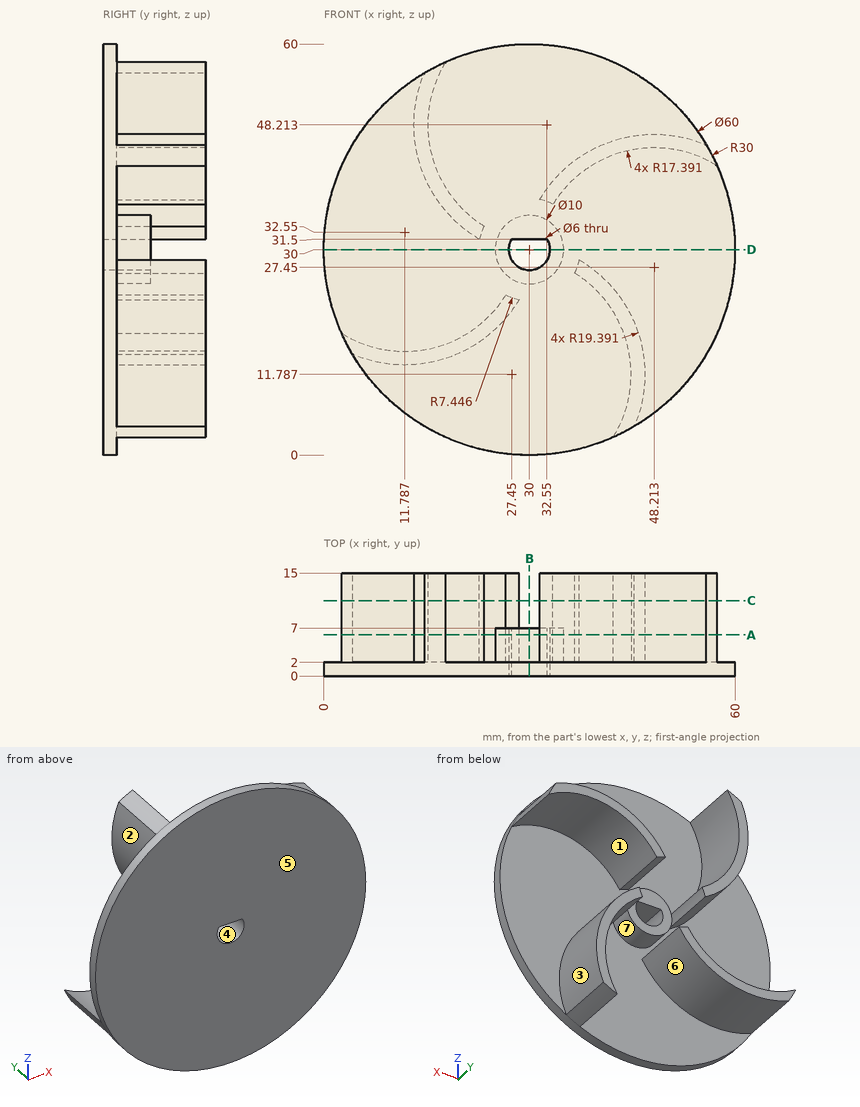
Answer from the drawing. Dimensions are ordinates in mm from the lowest x, y and z of the part. A direction names the side the tool comes from. Coordinates: 2 decimals unless noted, no trailing zeros. Write each loop counter-clockwise with the first axis right and the second up, starting at its lowest first coordinate (ties: lowest second). Pieces come first, ordered by that corner, then holes. Notation, with made-up numbers: (49, -24.75) - (94, -24.75) arc R18 ccw to (94, 1.25) - close; hole circle Ø7 at (-15, 36). An arc over 180 degrees is marked (long way). Return JSON: item names as keys, results as strings.
1. Consider line 1 along Z through (x, y) = (30, 4.75); line 2 along X through (y, z) = (4.75, 30); line 3 along X through (y, z) = (5.5, 28) (1 decimal). Determine where each line is inside the solid, lowest interval first.
Final values:
{"line 1": "25 to 27, 31.5 to 35", "line 2": "25 to 27, 33 to 35", "line 3": "25.4 to 27.8, 32.2 to 34.6, 37.2 to 38.1"}
2. Each of these flat-tipped pins is pushed along its axis until it touches: pin 1 Ø8 at (x, y) = (49.5, 7.5) entering from +Z; pin 2 Ø6 at (x, y) = (23, 12) entering from +Z (1 decimal); pin 3 Ø3 at (y, z) = (13, 16.5) entering from +X. Where does it stop, or does it pass through?
Final values:
{"pin 1": "z = 46.84", "pin 2": "z = 36.2", "pin 3": "x = 46.57"}
3. The part is cut by section D-D on z = 30. Determine the outline of the cut face in (x, y), then the cut area to 3 significant figures.
Final values:
{"outline": "(0, 0) - (27, 0) - (27, 7) - (25, 7) - (25, 2) - (0, 2) - close; (33, 0) - (60, 0) - (60, 2) - (35, 2) - (35, 7) - (33, 7) - close", "area": "128 mm^2"}
4. For a pull along X with two mould halves and no side action, classify the marked faces 1, 2, 3 and 4 as +X half, -X half, draft (parallel to the pull), parting line (faces both ways), or undercut.
Final values:
{"face 1": "undercut", "face 2": "-X half", "face 3": "+X half", "face 4": "undercut"}
5. The part is cut by section B-B on x = 30. Determine the outline of the cut face in (y, z).
Final values:
{"outline": "(0, 0) - (2, 0) - (2, 25) - (7, 25) - (7, 27) - (0, 27) - close; (0, 31.5) - (7, 31.5) - (7, 35) - (2, 35) - (2, 60) - (0, 60) - close"}
6. The part is cut by section C-C on y = 11. Determine the outline of the cut face in (x, z).
Final values:
{"outline": "(2.6, 17.78) arc R30 ccw to (4.19, 14.71) arc R19.39 ccw to (28.49, 22.71) arc R7.45 cw to (26.57, 23.39) arc R17.39 cw to start; (14.71, 55.81) arc R19.39 ccw to (22.71, 31.51) arc R7.45 cw to (23.39, 33.43) arc R17.39 cw to (17.78, 57.4) arc R30 ccw to start; (31.51, 37.29) arc R7.45 cw to (33.43, 36.61) arc R17.39 cw to (57.4, 42.22) arc R30 ccw to (55.81, 45.29) arc R19.39 ccw to start; (36.61, 26.57) arc R17.39 cw to (42.22, 2.6) arc R30 ccw to (45.29, 4.19) arc R19.39 ccw to (37.29, 28.49) arc R7.45 cw to start"}
7. The part is cut by section A-A on y = 6. Determine the outline of the cut face in (x, z).
Final values:
{"outline": "(2.6, 17.78) arc R30 ccw to (4.19, 14.71) arc R19.39 ccw to (28.49, 22.71) arc R7.45 cw to (26.57, 23.39) arc R17.39 cw to start; (14.71, 55.81) arc R19.39 ccw to (22.71, 31.51) arc R7.45 cw to (23.39, 33.43) arc R17.39 cw to (17.78, 57.4) arc R30 ccw to start; circle Ø10 at (30, 30); (31.51, 37.29) arc R7.45 cw to (33.43, 36.61) arc R17.39 cw to (57.4, 42.22) arc R30 ccw to (55.81, 45.29) arc R19.39 ccw to start; (36.61, 26.57) arc R17.39 cw to (42.22, 2.6) arc R30 ccw to (45.29, 4.19) arc R19.39 ccw to (37.29, 28.49) arc R7.45 cw to start; hole (27.4, 31.5) arc R3 ccw (long way) to (32.6, 31.5) - close"}
8. Which of the six approach directions +Z, -Z, +X, -X, +Y, -Y give full straight-line access (tool end or side, diameter ignored) to the marked faces 5, 6 and 7?
Final values:
{"face 5": "+Z, -Z, +X, -X, -Y", "face 6": "-Z, +Y", "face 7": "+Y"}
